from build123d import *

# Parameters (mm, degrees)
ESQUISSE1_W             = 218
ESQUISSE1_H             = 238
ESQUISSE1_W_2           = 20
ESQUISSE1_H_2           = 6
ESQUISSE1_W_3           = 30
ESQUISSE1_H_3           = 20
ESQUISSE1_W_4           = 15
ESQUISSE1_H_4           = 15
BOSS_EXTRU_1_DEPTH      = 6
ESQUISSE2_W             = 40
ESQUISSE2_H             = 25
ENL_V_MAT_EXTRU_1_DEPTH = 6
ESQUISSE3_W             = 20
ESQUISSE3_H             = 6
BOSS_EXTRU_3_DEPTH      = 6
ESQUISSE4_R             = 1.5
ENL_V_MAT_EXTRU_2_DEPTH = 6
ESQUISSE5_W             = 10
ESQUISSE5_H             = 244
BOSS_EXTRU_4_DEPTH      = 6
ESQUISSE6_W             = 20
ESQUISSE6_H             = 12
ENL_V_MAT_EXTRU_3_DEPTH = 6
ESQUISSE7_R             = 1.175
ENL_V_MAT_EXTRU_4_DEPTH = 7


with BuildPart() as part:
    # Esquisse1 → Boss.-Extru.1 (new body)
    with BuildSketch(Plane.XY):
        Rectangle(ESQUISSE1_W, ESQUISSE1_H)
        with Locations((-91, -13)):
            Rectangle(ESQUISSE1_W_2, ESQUISSE1_H_2, mode=Mode.SUBTRACT)
        with Locations((0, -13)):
            Rectangle(ESQUISSE1_W_2, ESQUISSE1_H_2, mode=Mode.SUBTRACT)
        with Locations((91, -13)):
            Rectangle(ESQUISSE1_W_2, ESQUISSE1_H_2, mode=Mode.SUBTRACT)
        with Locations((-66.5, 51)):
            Rectangle(ESQUISSE1_W_2, ESQUISSE1_H_2, mode=Mode.SUBTRACT)
        with Locations((66.5, 51)):
            Rectangle(ESQUISSE1_W_2, ESQUISSE1_H_2, mode=Mode.SUBTRACT)
        with Locations((45.5, -59)):
            Rectangle(ESQUISSE1_W_3, ESQUISSE1_H_3, mode=Mode.SUBTRACT)
        with Locations((65, 96)):
            Rectangle(ESQUISSE1_W_2, ESQUISSE1_H_2, mode=Mode.SUBTRACT)
        with Locations((95, 96)):
            Rectangle(ESQUISSE1_W_2, ESQUISSE1_H_2, mode=Mode.SUBTRACT)
        with Locations((31.5, 71.5)):
            Rectangle(ESQUISSE1_W_4, ESQUISSE1_H_4, mode=Mode.SUBTRACT)
    extrude(amount=BOSS_EXTRU_1_DEPTH)

    # Esquisse2 → Enlèv. mat.-Extru.1 (cut)
    with BuildSketch(Plane.XY.offset(6)):
        with Locations((-69, -106.5)):
            Rectangle(ESQUISSE2_W, ESQUISSE2_H)
        with Locations((69, -106.5)):
            Rectangle(ESQUISSE2_W, ESQUISSE2_H)
    extrude(amount=-ENL_V_MAT_EXTRU_1_DEPTH, mode=Mode.SUBTRACT)

    # Esquisse3 → Boss.-Extru.3 (add)
    with BuildSketch(Plane.XY.offset(6)):
        with Locations((-24, -122)):
            Rectangle(ESQUISSE3_W, ESQUISSE3_H)
        with Locations((24, -122)):
            Rectangle(ESQUISSE3_W, ESQUISSE3_H)
        with Locations((24, 122)):
            Rectangle(ESQUISSE3_W, ESQUISSE3_H)
        with Locations((99, 122)):
            Rectangle(ESQUISSE3_W, ESQUISSE3_H)
        with Locations((-24, 122)):
            Rectangle(ESQUISSE3_W, ESQUISSE3_H)
        with Locations((-99, 122)):
            Rectangle(ESQUISSE3_W, ESQUISSE3_H)
    extrude(amount=-BOSS_EXTRU_3_DEPTH)

    # Esquisse4 → Enlèv. mat.-Extru.2 (cut)
    with BuildSketch(Plane.XY.offset(6)):
        with Locations((-15, -13)):
            Circle(ESQUISSE4_R)
        with Locations((-76, -13)):
            Circle(ESQUISSE4_R)
        with Locations((80, 96)):
            Circle(ESQUISSE4_R)
        with Locations((51.5, 51)):
            Circle(ESQUISSE4_R)
        with Locations((76, -13)):
            Circle(ESQUISSE4_R)
        with Locations((15, -13)):
            Circle(ESQUISSE4_R)
        with Locations((-51.5, 51)):
            Circle(ESQUISSE4_R)
        with Locations((-99, 122)):
            Circle(ESQUISSE4_R)
        with Locations((-24, 122)):
            Circle(ESQUISSE4_R)
        with Locations((24, 122)):
            Circle(ESQUISSE4_R)
        with Locations((99, 122)):
            Circle(ESQUISSE4_R)
        with Locations((-91, -84)):
            Circle(ESQUISSE4_R)
        with Locations((-91, 44)):
            Circle(ESQUISSE4_R)
        with Locations((91, -84)):
            Circle(ESQUISSE4_R)
        with Locations((91, 44)):
            Circle(ESQUISSE4_R)
    extrude(amount=-ENL_V_MAT_EXTRU_2_DEPTH, mode=Mode.SUBTRACT)

    # Esquisse5 → Boss.-Extru.4 (add)
    with BuildSketch(Plane.XY.offset(6)):
        with Locations((-114, -3)):
            Rectangle(ESQUISSE5_W, ESQUISSE5_H)
        with Locations((114, -3)):
            Rectangle(ESQUISSE5_W, ESQUISSE5_H)
    extrude(amount=-BOSS_EXTRU_4_DEPTH)

    # Esquisse6 → Enlèv. mat.-Extru.3 (cut)
    with BuildSketch(Plane.XY.offset(6)):
        with Locations((99, -113)):
            Rectangle(ESQUISSE6_W, ESQUISSE6_H)
        with Locations((-99, -113)):
            Rectangle(ESQUISSE6_W, ESQUISSE6_H)
    extrude(amount=-ENL_V_MAT_EXTRU_3_DEPTH, mode=Mode.SUBTRACT)

    # Esquisse7 → Enlèv. mat.-Extru.4 (cut, through all)
    with BuildSketch(Plane.XY.offset(6)):
        with Locations((-8, 100.5)):
            Circle(ESQUISSE7_R)
        with Locations((8, 100.5)):
            Circle(ESQUISSE7_R)
        with Locations((-8, 84.5)):
            Circle(ESQUISSE7_R)
        with Locations((8, 84.5)):
            Circle(ESQUISSE7_R)
    extrude(amount=-ENL_V_MAT_EXTRU_4_DEPTH, mode=Mode.SUBTRACT)


solid = part.part
Model file for the job. Use its own axes, mm. A direction names the side the tool comes from. Give positions to 0.01 mm unless a question says otherwise; leave off trailing zeros. Order: outer loops, then holes, each group sorted by start corner. A loop starts at its lowest first (then second) coordinate and runs counter-clockwise, first axis right, second up. Notation, with made-up numbers: (-29.75, 6.25) - (-13.75, 6.25) arc R19 ccw to (-13.75, 18.25) - close; hole circle Ø11 at (4.5, 17.5). An arc over 180 degrees is marked (long way). One line per item, written item: value.
Item 1: Slice it at A-A (y = 69). List the corners of the cut face in (x, z), then the cut area to 3 significant figures.
Response values:
outline: (-119, 0) - (24, 0) - (24, 6) - (-119, 6) - close; (39, 0) - (119, 0) - (119, 6) - (39, 6) - close
area: 1,340 mm2
Item 2: Slice it at B-B (z = 2.6). Give the number of separate pieces and of enclosed holes in the cut face, then the cut area to 3 significant figures.
Response values:
separate pieces: 1
enclosed holes: 28
area: 53,200 mm2
Item 3: Pin check, flat tips, straight feed: pin 1 Ø1.8 at (x, z) = (66.5, 3) entering from +Y; pin 2 Ø3 at (x, z) = (-90.5, 3.5) entering from -Y; pin 3 Ø3 at (y, z) = (123, 4.5) entering from -X. Stop position of each tip, or through.
Response values:
pin 1: y = 119
pin 2: y = -107
pin 3: x = -109
Item 4: Wall check: line 1 (Y direction, x = 57, z = 4.85); line 2 (Y direction, x = -91, z = 4.05); line 3 (Y direction, x = 91, z = 2.8). Give the ranges that are in metal, low to high.
Response values:
line 1: -94 to -69, -49 to 48, 54 to 93, 99 to 119
line 2: -107 to -85.5, -82.5 to -16, -10 to 42.5, 45.5 to 125
line 3: -107 to -85.5, -82.5 to -16, -10 to 42.5, 45.5 to 93, 99 to 125
Item 5: Tool access for faces 5 (the flat face through (45, -49, 3)), 6 (the flat face through (-89, 122, 3)), 7 (the flat face through (49, -107, 3)): list every direction of +Z, -Z, +X, -X, +Y, -Y with a clear straight run to the whole face (end or side of a thin tool).
Response values:
face 5: +Z, -Z
face 6: +Z, -Z, +Y
face 7: +Z, -Z, -Y
Item 6: Two-plate mould, pull along X, no slides. Class faces 1 (the flat face through (24, 71, 3)), 2 (the flat face through (89, 122, 3)), 3 (the flat face through (119, -5, 3)), 4 (the flat face through (-114, 119, 3)): released by +X, released by -X, zero draft, split by the parting line, or undercut.
Response values:
face 1: undercut
face 2: undercut
face 3: released by +X
face 4: zero draft
